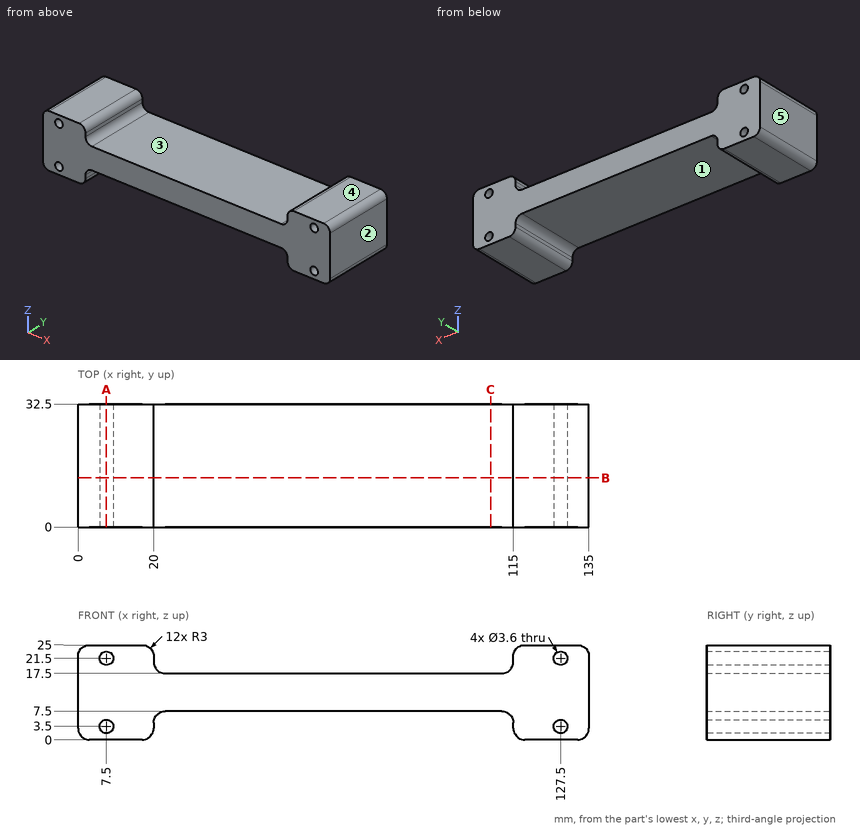
Drawing for the job (mm, zero at the part's lowest x, y, z). A direction names the side the tool comes from. Give positions to 0.01 mm unless a question says otherwise; leave off trailing zeros. Order: outer loops, then holes, each group sorted by start corner. A loop starts at its lowest first (then second) coordinate and runs counter-clockwise, first axis right, second up. Notation, with made-up numbers: M -19.75,78.25 L 18.25,78.25 A24 cw 18.25,114.25 Z; hole C 66,0.5 d3. An arc over 180 degrees is marked long. Write item = value, one per line. Start each with the question number.
(1) Two-plate mould, pull along X, no slides. Class the marked faces 3, 4 and 5: released by +X, released by -X, zero draft, split by the parting line, or undercut.
(2) Slice it at A-A on x = 7.5. Write the cut outline in (y, z), plus the area to 4 significant figures.
(3) Slice it at B-B on y = 13. Write the cut outline in (x, z), plus the area to 3 significant figures.
(4) Pin check, flat tips, straight feed: pin 1 Ø10 at (x, y) = (70, 9) entering from -Z; pin 2 Ø2 at (x, y) = (98, 7) entering from +Z. Stop position of each tip, or through.
(5) Which spindle directions (+Z, -Z, +X, -X, +Y, -Y) get a long thin tool onto all of the face, cutting with end or side? Do the marked faces 1 and 2. Say none if no direction does.
(6) Slice it at C-C on x = 109. Write the cut outline in (y, z).
(7) Probe L1, parallel to X at y = 25, z = 21.5; L2, parallel to Z at x = 127.5, y = 22; L3, parallel to Z at x = 7, y = 11. List the from-to ranges inside material, lowest first. Write a range as [from, to].
Responses:
q1.face_3 = undercut
q1.face_4 = zero draft
q1.face_5 = released by -X
q2.outline = M 0,0 L 32.5,0 L 32.5,1.7 L 0,1.7 Z; M 0,5.3 L 32.5,5.3 L 32.5,19.7 L 0,19.7 Z; M 0,23.3 L 32.5,23.3 L 32.5,25 L 0,25 Z
q2.area = 578.5 mm2
q3.outline = M 0,3 A3 ccw 3,0 L 17,0 A3 ccw 20,3 L 20,4.5 A3 cw 23,7.5 L 112,7.5 A3 cw 115,4.5 L 115,3 A3 ccw 118,0 L 132,0 A3 ccw 135,3 L 135,22 A3 ccw 132,25 L 118,25 A3 ccw 115,22 L 115,20.5 A3 cw 112,17.5 L 23,17.5 A3 cw 20,20.5 L 20,22 A3 ccw 17,25 L 3,25 A3 ccw 0,22 Z; hole C 7.5,3.5 d3.6; hole C 7.5,21.5 d3.6; hole C 127.5,3.5 d3.6; hole C 127.5,21.5 d3.6
q3.area = 1,900 mm2
q4.pin_1 = 7.5
q4.pin_2 = 17.5
q5.face_1 = -Z, +Y, -Y
q5.face_2 = +Z, -Z, +X, +Y, -Y
q6.outline = M 0,7.5 L 32.5,7.5 L 32.5,17.5 L 0,17.5 Z
q7.L1 = [0, 5.7], [9.3, 20], [115, 125.7], [129.3, 135]
q7.L2 = [0, 1.7], [5.3, 19.7], [23.3, 25]
q7.L3 = [0, 1.77], [5.23, 19.77], [23.23, 25]
